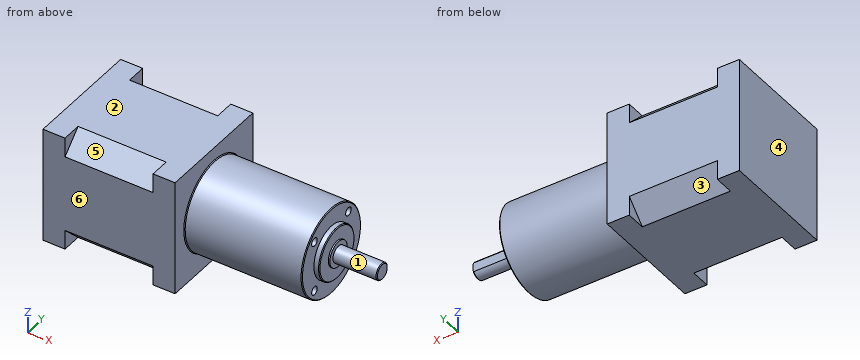
from build123d import *

# Parameters (mm, degrees)
SKETCH1_W           = 42
SKETCH1_H           = 42
BOSS_EXTRUDE1_DEPTH = 48
SKETCH2_R           = 16
BOSS_EXTRUDE2_DEPTH = 42.7
SKETCH7_W           = 16.587443852
SKETCH7_H           = 11.908554944
CUT_EXTRUDE1_DEPTH  = 2
CHAMFER1_SIZE       = 0.3
SKETCH8_R           = 1.5
CUT_EXTRUDE2_DEPTH  = 10
CUT_EXTRUDE3_DEPTH  = 32


with BuildPart() as part:
    # Sketch1 → Boss-Extrude1 (new body)
    with BuildSketch(Plane(origin=(0, 0, 0), x_dir=(0, 0, -1), z_dir=(1, 0, 0))):
        with Locations((21, 21)):
            Rectangle(SKETCH1_W, SKETCH1_H)
    extrude(amount=BOSS_EXTRUDE1_DEPTH)

    # Sketch2 → Boss-Extrude2 (add)
    with BuildSketch(Plane(origin=(48, 0, 0), x_dir=(0, 0, -1), z_dir=(1, 0, 0))):
        with Locations(Location((21, 21, 0), (0, 0, 180))):
            Circle(SKETCH2_R)
    extrude(amount=BOSS_EXTRUDE2_DEPTH)

    # Sketch5 → Revolve1 (revolve)
    with BuildSketch(Plane(origin=(0, 0, -21), x_dir=(-1, 0, 0), z_dir=(0, 0, -1)), mode=Mode.PRIVATE) as revolve1_sk:
        Polygon((-90.7, 30.5), (-92.7, 30.5), (-92.7, 25.65608714), (-93.252163767, 25.65608714), (-93.252163767, 24), (-109.2, 24), (-109.2, 21), (-90.7, 21), align=None)
    revolve(revolve1_sk.sketch.rotate(Axis((109.2, 21, -21), (-1, 0, 0)), 90), axis=Axis((109.2, 21, -21), (-1, 0, 0)))

    # Sketch7 → Cut-Extrude1 (cut)
    with BuildSketch(Plane(origin=(0, 23.5, 0), x_dir=(1, 0, 0), z_dir=(0, 1, 0))):
        with Locations((102.608605833, 20.527447563)):
            Rectangle(SKETCH7_W, SKETCH7_H)
    extrude(amount=CUT_EXTRUDE1_DEPTH, mode=Mode.SUBTRACT)

    # Chamfer1
    chamfer1_edges = [part.edges().sort_by_distance(p)[0] for p in [
        (48, 21, -37),
        (90.7, 21, -37),
        (92.7, 21, -11.5),
        (109.2, 18.356617963, -19.581362835),
    ]]
    chamfer(chamfer1_edges, length=CHAMFER1_SIZE)

    # Sketch8 → Cut-Extrude2 (cut)
    with BuildSketch(Plane(origin=(90.7, 0, 0), x_dir=(0, 0, -1), z_dir=(1, 0, 0))):
        with Locations((30.192388155, 30.192388155)):
            Circle(SKETCH8_R)
        with Locations((30.192388155, 11.807611845)):
            Circle(SKETCH8_R)
        with Locations((11.807611845, 11.807611845)):
            Circle(SKETCH8_R)
        with Locations((11.807611845, 30.192388155)):
            Circle(SKETCH8_R)
    extrude(amount=-CUT_EXTRUDE2_DEPTH, mode=Mode.SUBTRACT)

    # Sketch9 → Cut-Extrude3 (cut)
    with BuildSketch(Plane(origin=(40, 0, 0), x_dir=(0, 0, -1), z_dir=(1, 0, 0))):
        Polygon((0, 34.928932188), (7.071067812, 42), (0, 42), align=None)
        Polygon((0, 0), (7.071067812, 0), (0, 7.071067812), align=None)
        Polygon((42, 0), (42, 7.071067812), (34.928932188, 0), align=None)
        Polygon((34.928932188, 42), (42, 34.928932188), (42, 42), align=None)
    extrude(amount=-CUT_EXTRUDE3_DEPTH, mode=Mode.SUBTRACT)


solid = part.part
The listing builds one solid part. Answer for the finished solid, in the listing's coordinates (mm). Face numbers are marked on the shaded views. A direction names the side the tool comes from. Round coordinates to 2 decimals unless told otherwise and drop trailing zeros. Order: outer loops, then holes, each group sorted by start corner. A loop starts at its lowest first (then second) coordinate and runs counter-clockwise, first axis right, second up. Notation, with made-up numbers: (61, 50.25) -> (99, 50.25) arc R18 cw to (99, 57.25) -> close; hole circle Ø3 at (10, 74). An arc over 180 degrees is marked (long way). Write each question's results on one line, items separated by ' | '. Start each with the question number.
Q1. The mould has two halves that part along X. Classify the marked faces 4, 5 and 6: pulls with the +X half, pulls with the -X half, needs draft (parallel to the pull), parting line crosses it, or undercut.
Q2. Straight lines are drawn through the part: probe 1 along Z at (x, y) = (64, 18); probe 2 along X at (y, z) = (30, -37); probe 3 along X at (y, z) = (14, -12). For each, find the intervals that lie inside material, in ascending order. Write a range as from..to.
Q3. Each of these flat-tipped pins is pushed along its axis until it touches: pin 1 (2 mm diameter, centred on y = 37.5, z = -2.5, fed in from +X); pin 2 (5 mm diameter, centred on x = 53, z = -35.5, fed in from +Y); pin 3 (4 mm diameter, centred on x = 75.5, y = 8.5, fed in from -Z). Where does it stop, or does it pass through?
Q4. Which of the six approach directions +Z, -Z, +X, -X, +Y, -Y give full straight-line access (tool end or side, diameter ignored) to the marked faces 1, 2 and 3?
Q5. Find section A-A (x = 12.5). Determine the outline of the cut face in (y, z), then the cut area to 3 significant figures.
Q6. Find section C-C (y = 21). Determine the outline of the cut face in (x, z).
Q7. Find section D-D (x = 83). Determine the outline of the cut face in (y, z).
Worked answers:
1) face 4: pulls with the -X half | face 5: undercut | face 6: needs draft
2) probe 1: z = -36.72..-5.28 | probe 2: x = 0..48 | probe 3: x = 0..90.7
3) pin 1: stops at x = 48 | pin 2: stops at y = 31.58 | pin 3: stops at z = -33.07
4) face 1: +X | face 2: +Z, +X, -X, +Y, -Y | face 3: -Z, +Y
5) outline: (0, -34.93) -> (7.07, -42) -> (34.93, -42) -> (42, -34.93) -> (42, -7.07) -> (34.93, 0) -> (7.07, 0) -> (0, -7.07) -> close | area: 1,660 mm2
6) outline: (0, -42) -> (48, -42) -> (48, -37.3) -> (48.3, -37) -> (90.4, -37) -> (90.7, -36.7) -> (90.7, -30.5) -> (92.4, -30.5) -> (92.7, -30.2) -> (92.7, -25.66) -> (93.25, -25.66) -> (93.25, -24) -> (108.9, -24) -> (109.2, -23.7) -> (109.2, -18.3) -> (108.9, -18) -> (93.25, -18) -> (93.25, -16.34) -> (92.7, -16.34) -> (92.7, -11.8) -> (92.4, -11.5) -> (90.7, -11.5) -> (90.7, -5.3) -> (90.4, -5) -> (48.3, -5) -> (48, -4.7) -> (48, 0) -> (0, 0) -> close
7) outline: circle Ø32 at (21, -21); hole circle Ø3 at (11.81, -30.19); hole circle Ø3 at (11.81, -11.81); hole circle Ø3 at (30.19, -30.19); hole circle Ø3 at (30.19, -11.81)
